```python
from build123d import *

# Parameters (mm, degrees)
F1_DEPTH = 7.5
F2_R     = 1
F4_DEPTH = 5


with BuildPart() as f1:
    # F0 (on Front) → F1 (new body, symmetric)
    with BuildSketch(Plane.XZ):
        with BuildLine():
            Line((30, 0), (1, 0))
            ThreePointArc((1, 0), (0.2928932188, -0.2928932188), (0, -1))
            Line((0, -1), (0, -56))
            ThreePointArc((0, -56), (0.2928932188, -56.7071067812), (1, -57))
            Line((1, -57), (30, -57))
            ThreePointArc((30, -57), (30.7071067812, -56.7071067812), (31, -56))
            Line((31, -56), (31, -1))
            ThreePointArc((31, -1), (30.7071067812, -0.2928932188), (30, 0))
        make_face()
    extrude(amount=F1_DEPTH, both=True)

    # F2
    f2_edges = [f1.edges().sort_by_distance(p)[0] for p in [
        (15.5, -7.5, 0),
        (0.292893, -7.5, -0.292893),
        (0, -7.5, -28.5),
        (0.292893, -7.5, -56.707107),
        (15.5, -7.5, -57),
        (30.707107, -7.5, -56.707107),
        (31, -7.5, -28.5),
        (30.707107, -7.5, -0.292893),
        (15.5, 7.5, 0),
        (0.292893, 7.5, -0.292893),
        (0, 7.5, -28.5),
        (0.292893, 7.5, -56.707107),
        (15.5, 7.5, -57),
        (30.707107, 7.5, -56.707107),
        (31, 7.5, -28.5),
        (30.707107, 7.5, -0.292893),
    ]]
    fillet(f2_edges, radius=F2_R)

    # F3 (on Front) → F4 (join, symmetric)
    with BuildSketch(Plane.XZ):
        Polygon((29, 0), (30, -1), (34.2426406871, 3.2426406871), (33.2426406871, 4.2426406871), align=None)
    extrude(amount=F4_DEPTH, both=True)


solid = f1.part
```
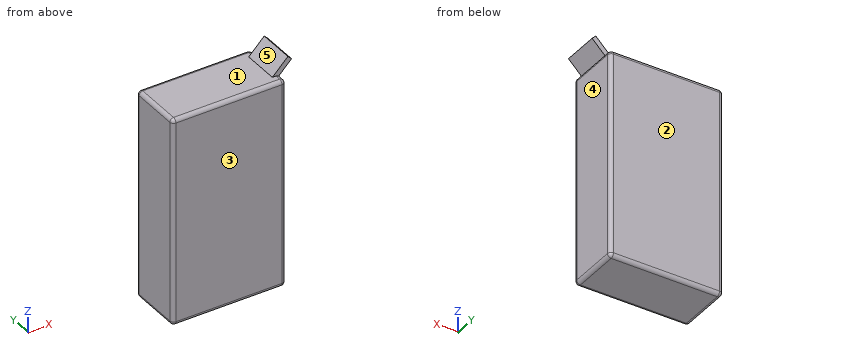
Design review of the part built by this model. Coordinates are the model's own, in mm. Face numbers are marked on the shaded views. A direction names the side the tool comes from. Round coordinates to 2 decimals unless told otherwise and drop trailing zeros. Write each loop counter-clockwise with the first axis right and the second up, starting at its lowest first coordinate (ties: lowest second). Pieces come first, ordered by that corner, then holes.
Item 1: We need section C-C on z = -7. Write out the cut boundary in (x, y), and give its area (3 significant figures).
Item 2: Clearance check with flat-ended pins moving along their axes: pin 1 Ø3 at (y, z) = (3, -35.5) entering from +X; pin 2 Ø5 at (x, z) = (32.5, 1.5) entering from +Y; pin 3 Ø4 at (x, y) = (22.5, 3) entering from +Z. State where each tip first meets the part, or that it passes through.
Item 3: We need section B-B on x = 22. Write out the cut boundary in (y, z), and give its area (3 significant figures).
Item 4: For probe 1 along X at (y, z) = (-1.75, -47); probe 2 along Z at (x, y) = (16.5, -4.25); probe 3 along X at (y, z) = (7, -41), list the stretches that pass through material, from the lowest coordinate up.
Item 5: We need section A-A on y = -4. Write out the cut boundary in (x, z), and give its area (3 significant figures).
Item 6: The part is to be moulded in two halves that separate along Y. For the marked faces 1, 2 and 3, say which applies: +Y half, -Y half, draft (parallel to the pull), parting line (faces both ways), or undercut.
Item 7: For the marked faces 4 and 5, list the 3-axis set-ups (+Z, -Z, +X, -X, +Y, -Y) from which the entire face can be reached by the end or side of a thin tool; tool diameter is ignored.
Returned:
1. outline: (0, -6.5) arc R1 ccw to (1, -7.5) - (30, -7.5) arc R1 ccw to (31, -6.5) - (31, 6.5) arc R1 ccw to (30, 7.5) - (1, 7.5) arc R1 ccw to (0, 6.5) - close
1. area: 464 mm2
2. pin 1: stops at x = 31
2. pin 2: stops at y = 5
2. pin 3: stops at z = 0
3. outline: (-7.5, -56) arc R1 ccw to (-6.5, -57) - (6.5, -57) arc R1 ccw to (7.5, -56) - (7.5, -1) arc R1 ccw to (6.5, 0) - (-6.5, 0) arc R1 ccw to (-7.5, -1) - close
3. area: 854 mm2
4. probe 1: x = 0 to 31
4. probe 2: z = -57 to 0
4. probe 3: x = 0.13 to 30.87
5. outline: (0, -56) arc R1 ccw to (1, -57) - (30, -57) arc R1 ccw to (31, -56) - (31, -1) arc R1 ccw to (30.71, -0.29) - (34.24, 3.24) - (33.24, 4.24) - (29, 0) - (1, 0) arc R1 ccw to (0, -1) - close
5. area: 1,770 mm2
6. face 1: draft
6. face 2: +Y half
6. face 3: -Y half
7. face 4: -Z, +X, +Y, -Y
7. face 5: +Z, -X, +Y, -Y
